Read the model definition and answer for the solid it produces. Units are mm, in the model's axes. Face numbers are marked on the shaded views. A direction names the side the tool comes from. Coordinates: 2 decimals unless noted, no trailing zeros. Order: outer loops, then holes, each group sorted by start corner. A loop starts at its lowest first (then second) coordinate and runs counter-clockwise, first axis right, second up. Notation, with made-up numbers: (-39.5, 23.5) -> (-12.5, 23.5) arc R23 cw to (-12.5, 50.5) -> close; hole circle Ø6 at (-24.75, -29). An arc over 180 degrees is marked (long way). Use CSV: the item, a comma, the result in double quotes.
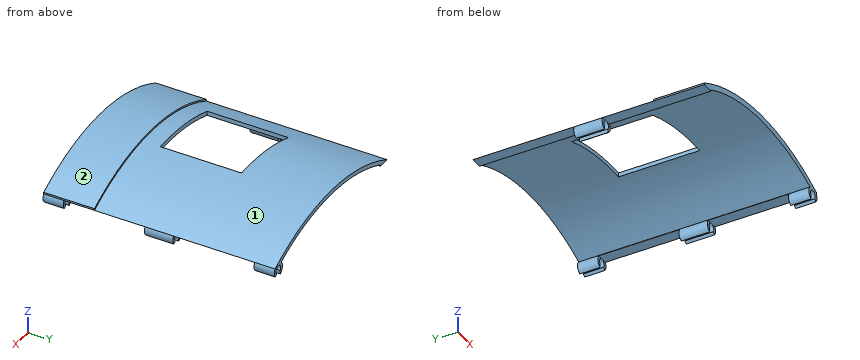
```python
from build123d import *

# Parameters (mm, degrees)
EXTRUDE_1_DEPTH     = 114
EXTRUDE_2_DEPTH     = 25
SKETCH_4_W          = 16.237843285
SKETCH_4_H          = 40
SKETCH_4_W_2        = 18.842025699
SKETCH_4_H_2        = 50
SKETCH_4_W_3        = 19.914336105
CUT_EXTRUDE_1_DEPTH = 20
SKETCH_5_W          = 40
SKETCH_5_H          = 40
CUT_EXTRUDE_2_DEPTH = 20


with BuildPart() as part:
    # 草图1 → 凸台-拉伸1 (new body)
    with BuildSketch(Plane(origin=(0, 0, 0), x_dir=(1, 0, 0), z_dir=(0, 1, 0))):
        with BuildLine():
            Line((90.5, 3.322875656), (90.5, 5.16227766))
            ThreePointArc((90.5, 5.16227766), (88.549473904, 2.586404006), (89.539550125, -0.489214015))
            ThreePointArc((89.539550125, -0.489214015), (47, -10.203390265), (4.460449875, -0.489214015))
            ThreePointArc((4.460449875, -0.489214015), (5.450526096, 2.586404006), (3.5, 5.16227766))
            Line((3.5, 5.16227766), (3.5, 3.322875656))
            ThreePointArc((3.5, 3.322875656), (2, 0), (0.5, 3.322875656))
            Line((0.5, 3.322875656), (0.5, 5.16227766))
            ThreePointArc((0.5, 5.16227766), (-1.382526963, 2.89917259), (-0.872281323, 0))
            ThreePointArc((-0.872281323, 0), (47, -12.203390265), (94.872281323, 0))
            ThreePointArc((94.872281323, 0), (95.494266967, 2.200245764), (94.625, 4.315032397))
            Line((94.625, 4.315032397), (93.5, 3.322875656))
            ThreePointArc((93.5, 3.322875656), (92, 0), (90.5, 3.322875656))
        make_face()
    extrude(amount=EXTRUDE_1_DEPTH)

    # 草图3 → 凸台-拉伸2 (add)
    with BuildSketch(Plane.XZ):
        with BuildLine():
            Line((-0.872281323, 0), (-0.872281323, 0.853303863))
            ThreePointArc((-0.872281323, 0.853303863), (47, 12.953390265), (94.872281323, 0.853303863))
            Line((94.872281323, 0.853303863), (94.872281323, 0))
            ThreePointArc((94.872281323, 0), (47, 12.203390265), (-0.872281323, 0))
        make_face()
    extrude(amount=-EXTRUDE_2_DEPTH)

    # 草图4 → 切除-拉伸1 (cut)
    with BuildSketch(Plane.XY):
        with Locations((92.649785841, 84)):
            Rectangle(SKETCH_4_W, SKETCH_4_H)
        with Locations((92.649785841, 30)):
            Rectangle(SKETCH_4_W, SKETCH_4_H)
        with Locations((0.967246157, 89)):
            Rectangle(SKETCH_4_W_2, SKETCH_4_H_2)
        with Locations((1.50340136, 25)):
            Rectangle(SKETCH_4_W_3, SKETCH_4_H_2)
    extrude(amount=-CUT_EXTRUDE_1_DEPTH, mode=Mode.SUBTRACT)

    # 草图5 → 切除-拉伸2 (cut)
    with BuildSketch(Plane.XY):
        with Locations((34.127718677, 54)):
            Rectangle(SKETCH_5_W, SKETCH_5_H)
    extrude(amount=CUT_EXTRUDE_2_DEPTH, mode=Mode.SUBTRACT)


solid = part.part
```
Item 1: Find section C-C, the plane x = 32.5. Give the vertices of the cut face in (y, z), then the cut area to 3 significant figures.
Return value:
outline,"(0, 9.12) -> (34, 9.12) -> (34, 11.15) -> (25, 11.15) -> (25, 11.9) -> (0, 11.9) -> close; (74, 9.12) -> (114, 9.12) -> (114, 11.15) -> (74, 11.15) -> close"
area,"169 mm^2"
Item 2: Find section A-A, the plane y = 52.5. Give the vertices of the cut face in (x, z) (3 decimals).
Return value:
outline,"(-0.872, 0) arc R3.5 ccw to (0.5, -5.162) -> (0.5, -3.323) arc R2 cw (long way) to (3.5, -3.323) -> (3.5, -5.162) arc R3.5 ccw to (4.46, 0.489) arc R98 cw to (14.128, 4.526) -> (14.128, 6.646) arc R100 ccw to start; (54.128, 9.944) arc R98 cw to (89.54, 0.489) arc R3.5 ccw to (90.5, -5.162) -> (90.5, -3.323) arc R2 cw (long way) to (93.5, -3.323) -> (94.625, -4.315) arc R3.5 ccw to (94.872, 0) arc R100 ccw to (54.128, 11.949) -> close"
Item 3: Find section D-D, the plane y = 28.5. Give the vertices of the cut face in (x, z).
Return value:
outline,"(-0.87, 0) -> (4.87, 0) arc R3.5 ccw to (4.46, 0.49) arc R98 cw to (89.54, 0.49) arc R3.5 ccw to (89.13, 0) -> (94.87, 0) arc R100 ccw to start"
Item 4: Straight lines are drawn through the part: line 1 along X through (y, z) = (60.5, -2); line 2 along X through (y, z) = (8, -2); line 3 along Y through (x, z) = (5, 3.5). For each, find the intervals that lie inside material, in ascending order.
Return value:
line 1,"x = -1.5 to 0, 4 to 5.5, 88.5 to 90, 94 to 95.5"
line 2,"x = 88.5 to 90, 94 to 95.5"
line 3,"y = 0 to 25"
Item 5: A tool of negligible diameter and unlimited length cuts with its end or side. For the marked faces 1 and 2, from which of +Z, -Z, +X, -X, +Y, -Y can it reach the whole face along a straight path? Write none if from no direction.
Return value:
face 1,"+Z, +Y"
face 2,"+Z, +Y, -Y"
Item 6: Find section B-B, the plane z = -2. Give the number of separate pieces and of enclosed holes in the cut face, then the cut area to 3 significant figures.
Return value:
separate pieces,"8"
enclosed holes,"0"
area,"144 mm^2"
Item 7: Each of these flat-tipped pins is pushed along its axis until it touches: P1, Ø3, axis at y = 60.5, z = 2.5, coming from the -X side; P2, Ø1, axis at y = 46.5, z = 11, coming from the -X side; P3, Ø4, axis at x = 0.5, z = -2.5, coming from the +Y side. Where does it stop, or does it pass through?
Return value:
P1,"stops at x = 1.01"
P2,"stops at x = 54.13"
P3,"stops at y = 64"
